Build history of the part. All positions in model axes, mm. A direction names the side the tool comes from. Round coordinates to 2 decimals unless told otherwise and drop trailing zeros. Write each loop counter-clockwise with the first axis right and the second up, starting at its lowest first coordinate (ties: lowest second). Pieces come first, ordered by that corner, then holes.
Item 1: Wall check: probe 1 along X at (y, z) = (1.2, -10.75) (3 decimals); probe 2 along Z at (x, y) = (6.25, 0.75); probe 3 along X at (y, z) = (1.75, -1) (3 decimals). Give the ranges that are in metal, low to high.
Item 2: Mould opens along X. For faces 1 (the flat face through (10, 1, -5.3)), 2 (the flat face through (4.425, 1, -1)) say: +X half, -X half, draft (parallel to the pull), parting line (faces both ways), or undercut.
Item 3: Band-saw the part on C-C, the plane z = -1.75. Write the cut outline in (x, y), then the cut area to 3 significant figures.
Item 4: Band-saw the part on B-B, the plane x = 12.25. Write the cut outline in (y, z).
Item 5: Band-saw the part on D-D, the plane x = 2. Write the cut outline in (y, z), then the cut area to 3 significant figures.
Item 6: 3-axis set-ups, long thin cutter, end or side, ignore diameter. For faces 3 (the flat face through (12, 1, -10.6)), 4 (the flat face through (7, 2, -6)), 5 (the flat face through (2.925, 1, -6)): which of +Z, -Z, +X, -X, +Y, -Y reach the whole face in a straight line?
Item 7: Band-saw the part on A-A, the plane y = 0.7. Count the separate pieces of the cut face and the enclosed holes in it, then the cut area to 3 significant figures.
```python
from build123d import *

# Parameters (mm, degrees)
SKETCH1_W           = 13.2
SKETCH1_H           = 12.1
BOSS_EXTRUDE1_DEPTH = 3
SKETCH2_W           = 1.5
SKETCH2_H           = 1.5
BOSS_EXTRUDE2_DEPTH = 2
FILLET1_R           = 0.5


with BuildPart() as part:
    # Sketch1 → Boss-Extrude1 (new body)
    with BuildSketch(Plane(origin=(0, 0, 0), x_dir=(1, 0, 0), z_dir=(0, 1, 0))):
        with Locations((6.6, 6.05)):
            Rectangle(SKETCH1_W, SKETCH1_H)
    extrude(amount=-BOSS_EXTRUDE1_DEPTH)

    # Sketch2 → Boss-Extrude2 (add)
    with BuildSketch(Plane(origin=(0, 0, 0), x_dir=(1, 0, 0), z_dir=(0, 1, 0))):
        with Locations((3.675, 11.35)):
            Rectangle(SKETCH2_W, SKETCH2_H)
        with Locations((0.75, 11.35)):
            Rectangle(SKETCH2_W, SKETCH2_H)
        with Locations((6.6, 11.35)):
            Rectangle(SKETCH2_W, SKETCH2_H)
        with Locations((9.525, 11.35)):
            Rectangle(SKETCH2_W, SKETCH2_H)
        with Locations((12.45, 11.35)):
            Rectangle(SKETCH2_W, SKETCH2_H)
        with Locations((3.675, 8.7)):
            Rectangle(SKETCH2_W, SKETCH2_H)
        with Locations((6.6, 8.7)):
            Rectangle(SKETCH2_W, SKETCH2_H)
        with Locations((9.525, 8.7)):
            Rectangle(SKETCH2_W, SKETCH2_H)
        with Locations((12.45, 8.7)):
            Rectangle(SKETCH2_W, SKETCH2_H)
        with Locations((3.675, 6.05)):
            Rectangle(SKETCH2_W, SKETCH2_H)
        with Locations((6.6, 6.05)):
            Rectangle(SKETCH2_W, SKETCH2_H)
        with Locations((9.525, 6.05)):
            Rectangle(SKETCH2_W, SKETCH2_H)
        with Locations((12.45, 6.05)):
            Rectangle(SKETCH2_W, SKETCH2_H)
        with Locations((3.675, 3.4)):
            Rectangle(SKETCH2_W, SKETCH2_H)
        with Locations((6.6, 3.4)):
            Rectangle(SKETCH2_W, SKETCH2_H)
        with Locations((9.525, 3.4)):
            Rectangle(SKETCH2_W, SKETCH2_H)
        with Locations((12.45, 3.4)):
            Rectangle(SKETCH2_W, SKETCH2_H)
        with Locations((3.675, 0.75)):
            Rectangle(SKETCH2_W, SKETCH2_H)
        with Locations((6.6, 0.75)):
            Rectangle(SKETCH2_W, SKETCH2_H)
        with Locations((9.525, 0.75)):
            Rectangle(SKETCH2_W, SKETCH2_H)
        with Locations((12.45, 0.75)):
            Rectangle(SKETCH2_W, SKETCH2_H)
        with Locations((0.75, 8.7)):
            Rectangle(SKETCH2_W, SKETCH2_H)
        with Locations((0.75, 6.05)):
            Rectangle(SKETCH2_W, SKETCH2_H)
        with Locations((0.75, 3.4)):
            Rectangle(SKETCH2_W, SKETCH2_H)
        with Locations((0.75, 0.75)):
            Rectangle(SKETCH2_W, SKETCH2_H)
    extrude(amount=BOSS_EXTRUDE2_DEPTH)

    # Fillet1
    fillet1_edges = [part.edges().sort_by_distance(p)[0] for p in [
        (13.2, 2, -8.7),
        (13.2, 2, -6.05),
        (0, 2, -11.35),
        (0.75, 2, -12.1),
        (13.2, 2, -3.4),
        (3.675, 2, 0),
        (6.6, 2, 0),
        (9.525, 2, 0),
        (12.45, 2, 0),
        (13.2, 2, -0.75),
        (0, 2, -8.7),
        (0, 2, -6.05),
        (0, 2, -3.4),
        (0, 2, -0.75),
        (0.75, 2, 0),
        (3.675, 2, -12.1),
        (6.6, 2, -12.1),
        (9.525, 2, -12.1),
        (12.45, 2, -12.1),
        (13.2, 2, -11.35),
        (0, -0.5, -12.1),
        (13.2, -0.5, -12.1),
        (13.2, -0.5, 0),
        (0, -0.5, 0),
    ]]
    fillet(fillet1_edges, radius=FILLET1_R)


solid = part.part
```
Results:
1. probe 1: x = 0 to 1.5, 2.925 to 4.425, 5.85 to 7.35, 8.775 to 10.275, 11.7 to 13.2
1. probe 2: z = -12.1 to -10.6, -9.45 to -7.95, -6.8 to -5.3, -4.15 to -2.65, -1.5 to 0
1. probe 3: x = 0.067 to 1.5, 2.925 to 4.425, 5.85 to 7.35, 8.775 to 10.275, 11.7 to 13.133
2. face 1: draft
2. face 2: undercut
3. outline: (0, -3) - (13.2, -3) - (13.2, 0) - (0, 0) - close
3. area: 39.6 mm2
4. outline: (-3, -12.1) - (1.5, -12.1) arc R0.5 ccw to (2, -11.6) - (2, -10.6) - (0, -10.6) - (0, -9.45) - (2, -9.45) - (2, -7.95) - (0, -7.95) - (0, -6.8) - (2, -6.8) - (2, -5.3) - (0, -5.3) - (0, -4.15) - (2, -4.15) - (2, -2.65) - (0, -2.65) - (0, -1.5) - (2, -1.5) - (2, -0.5) arc R0.5 ccw to (1.5, 0) - (-3, 0) - close
5. outline: (-3, -12.1) - (0, -12.1) - (0, 0) - (-3, 0) - close
5. area: 36.3 mm2
6. face 3: +X, -X, +Y
6. face 4: +Z, -Z, +X, -X, +Y
6. face 5: +Z, -Z, +Y
7. separate pieces: 25
7. enclosed holes: 0
7. area: 56.0 mm2
